Build history of the part. All positions in model axes, mm. Face numbers are marked on the shaded views. Coordinates: 2 decimals unless noted, no trailing zeros. Write each loop counter-clockwise with the first axis right and the second up, starting at its lowest first coordinate (ties: lowest second). Pieces come first, ordered by that corner, then holes.
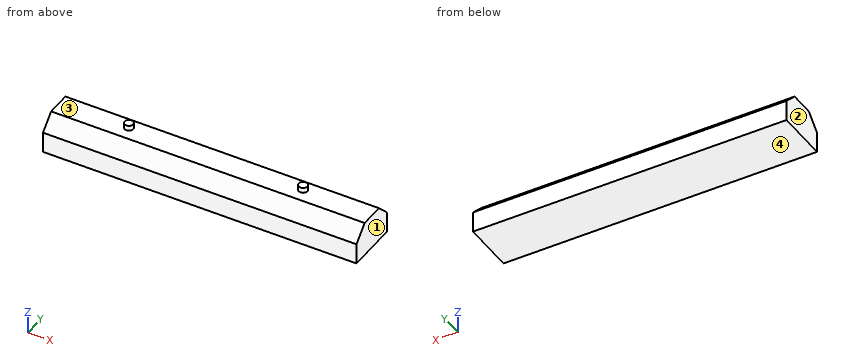
```python
from build123d import *

# Parameters (mm, degrees)
F0_W     = 3.81
F0_H     = 2.54
F1_DEPTH = 22.86
F2_SIZE  = 1.016
F3_R     = 0.309594
F3_R_2   = 0.3175
F4_DEPTH = 0.381


with BuildPart() as f1:
    # F0 (on Right) → F1 (new body)
    with BuildSketch(Plane.YZ):
        with Locations((1.905, 1.27)):
            Rectangle(F0_W, F0_H)
    extrude(amount=F1_DEPTH)

    # F2
    f2_edges = [f1.edges().sort_by_distance(p)[0] for p in [
        (11.43, 0, 2.54),
        (11.43, 3.81, 2.54),
    ]]
    chamfer(f2_edges, length=F2_SIZE)

    # F3 (on face) → F4 (join)
    with BuildSketch(Plane.XY.offset(2.54)):
        with Locations((5.08, 2.032)):
            Circle(F3_R)
        with Locations((17.78, 2.032)):
            Circle(F3_R_2)
    extrude(amount=F4_DEPTH)


solid = f1.part
```
1. Saw through at D-D on y = 0.5. List the corners of the cut face in (x, z), plus the area to 3 significant figures.
Computed values:
outline: (0, 0) - (22.86, 0) - (22.86, 2.02) - (0, 2.02) - close
area: 46.3 mm2
2. Mould opens along X. For the marked faces 1, 2, 3 and 4 say: +X half, -X half, draft (parallel to the pull), parting line (faces both ways), or undercut.
Computed values:
face 1: +X half
face 2: -X half
face 3: undercut
face 4: draft
3. Saw through at A-A on x = 17.78. List the corners of the cut face in (y, z), plus the area to 3 significant figures.
Computed values:
outline: (0, 0) - (3.81, 0) - (3.81, 1.52) - (2.79, 2.54) - (2.35, 2.54) - (2.35, 2.92) - (1.71, 2.92) - (1.71, 2.54) - (1.02, 2.54) - (0, 1.52) - close
area: 8.89 mm2
4. Flat gauge pin, fed straight in: pin 1 (1.5 mm diameter, centred on x = 8.5, y = 3.5, fed in from +Z). Where does the tip first touch, or does it go through?
Computed values:
pin 1: stops at z = 2.54
5. Saw through at B-B on y = 1.4. List the corners of the cut face in (x, z), plus the area to 3 significant figures.
Computed values:
outline: (0, 0) - (22.86, 0) - (22.86, 2.54) - (0, 2.54) - close
area: 58.1 mm2
6. Probe line 1 along Z through (x, y) = (10.5, 1.5); line 2 along Y through (x, z) = (10.5, 2.1); line 3 along Y through (x, z) = (20.5, 2.2). List the from-to ranges inside material, lowest first.
Computed values:
line 1: z = 0 to 2.54
line 2: y = 0.58 to 3.23
line 3: y = 0.68 to 3.13
7. Saw through at C-C on x = 5.08. List the corners of the cut face in (y, z).
Computed values:
outline: (0, 0) - (3.81, 0) - (3.81, 1.52) - (2.79, 2.54) - (2.34, 2.54) - (2.34, 2.92) - (1.72, 2.92) - (1.72, 2.54) - (1.02, 2.54) - (0, 1.52) - close
